Job drawing, mm, ordinate dimensions from the low corner. One solid piece. A direction names the side the tool comes from. Round coordinates to 2 decimals unless told otherwise and drop trailing zeros. Write each loop counter-clockwise with the first axis right and the second up, starting at its lowest first coordinate (ties: lowest second). Pieces come first, ordered by that corner, then holes. Notation, with made-up numbers: M -23,-26.5 L 10,-26.5 A32 cw 10,3.5 Z; hole C 61,-27.5 d4. An arc over 180 degrees is marked long. Answer as a JSON object with one key per item and string values. Group by question number.
1. Band-saw the part on C-C, the plane x = 29.5. Write the cut outline in (y, z), plus the area to 3 significant figures.
2. Band-saw the part on A-A, the plane x = 2.35. Write the cut outline in (y, z), plus the area to 3 significant figures.
3. Drop flat-ended pins along their axis: pin 1 (4 mm diameter, centred on y = 9.5, z = 5.5, fed in from -X); pin 2 (1.8 mm diameter, centred on x = 2.35, z = 6.15, fed in from -Y); pin 3 (12 mm diameter, centred on x = 3.5, y = 13.5, fed in from -Z); pin 4 (2.5 mm diameter, centred on x = 2, z = 4, fed in from -Y). Give the stop position or say it passes through.
4. Drill centre lines: line 1 (Z direction, x = 29.75, y = 20.15); line 2 (Y direction, x = 29, z = 9.5); line 3 (X direction, y = 14.5, z = 6.75). Where is each one in solid material? Low to high. Write a range as from..to.
5. Which spindle directions (+Z, -Z, +X, -X, +Y, -Y) get a long thin tool onto all of the face, cutting with end or side? Do the marked faces 1, 2, 3 and 4. Say none if no direction does.
6. Band-saw the part on D-D, the plane y = 10.5. Write the cut outline in (x, z).
7. Band-saw the part on B-B, the plane z = 4. Write the cut outline in (x, y).
8. Two-plate mould, pull along X, no slides. Class the marked faces 5, 6 and 7: +X half, -X half, draft (parallel to the pull), parting line (faces both ways), or undercut.
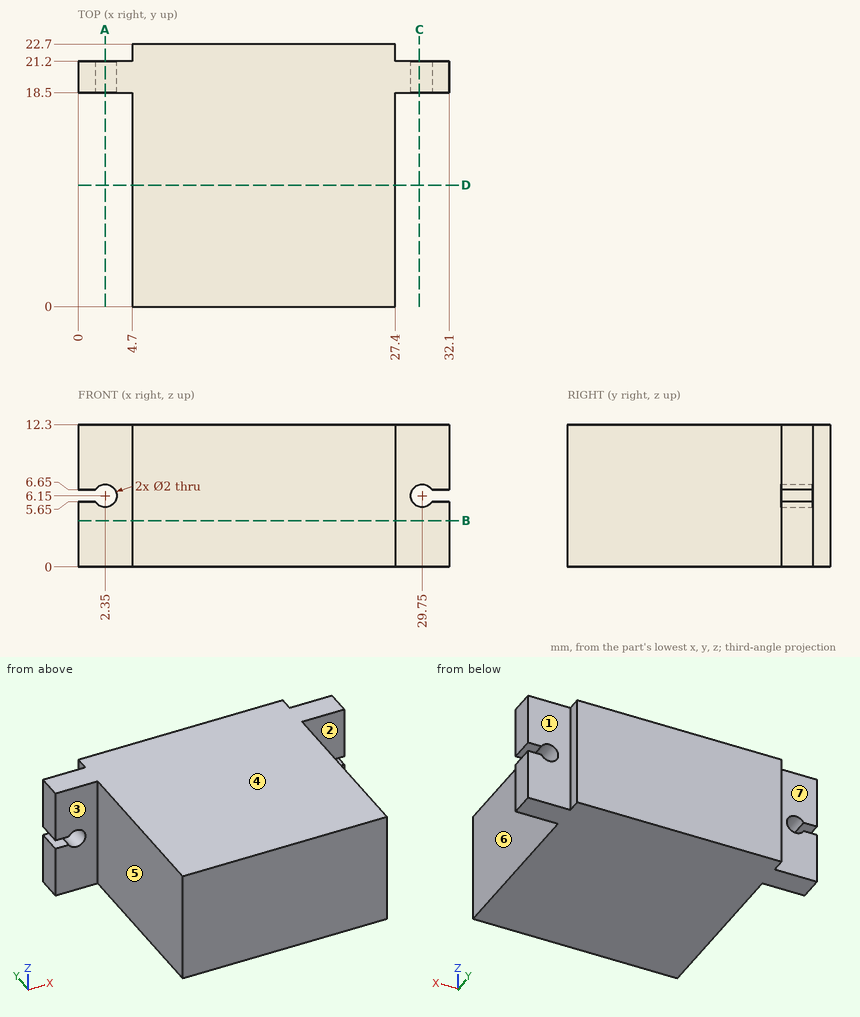
Worked answers:
{
 "1": {"outline": "M 18.5,0 L 21.2,0 L 21.2,5.18 L 18.5,5.18 Z; M 18.5,7.12 L 21.2,7.12 L 21.2,12.3 L 18.5,12.3 Z", "area": "28.0 mm^2"},
 "2": {"outline": "M 18.5,0 L 21.2,0 L 21.2,5.15 L 18.5,5.15 Z; M 18.5,7.15 L 21.2,7.15 L 21.2,12.3 L 18.5,12.3 Z", "area": "27.8 mm^2"},
 "3": {"pin 1": "stops at x = 4.7", "pin 2": "passes through", "pin 3": "stops at z = 0", "pin 4": "stops at y = 18.5"},
 "4": {"line 1": "z = 0..5.15, 7.15..12.3", "line 2": "y = 18.5..21.2", "line 3": "x = 4.7..27.4"},
 "5": {"face 1": "+Z, -Z, +X, +Y", "face 2": "+Z, -Z, +X, -Y", "face 3": "+Z, -Z, -X, -Y", "face 4": "+Z, +X, -X, +Y, -Y"},
 "6": {"outline": "M 4.7,0 L 27.4,0 L 27.4,12.3 L 4.7,12.3 Z"},
 "7": {"outline": "M 0,18.5 L 4.7,18.5 L 4.7,0 L 27.4,0 L 27.4,18.5 L 32.1,18.5 L 32.1,21.2 L 27.4,21.2 L 27.4,22.7 L 4.7,22.7 L 4.7,21.2 L 0,21.2 Z"},
 "8": {"face 5": "-X half", "face 6": "+X half", "face 7": "draft"}
}
